Work out the finished part from the listing and answer in its coordinate system (mm). Face numbers are marked on the shaded views. A direction names the side the tool comes from. Round coordinates to 2 decimals unless told otherwise and drop trailing zeros. Write each loop counter-clockwise with the first axis right and the second up, starting at its lowest first coordinate (ties: lowest second). Pieces come first, ordered by that corner, then holes. Notation, with made-up numbers: M -21,53.25 L 5,53.25 A9 ccw 5,63.25 Z; hole C -26.5,48 d9. An arc over 180 degrees is marked long. One line per item, written item: value. Start each with the question number.
Q1. A tool of negligible diameter and unlimited length cuts with its end or side. For the marked faces 4 and 5, from which of +Z, -Z, +X, -X, +Y, -Y can it reach the whole face along a straight path? Write none if from no direction.
Q2. The mould has two halves that part along Y. Classify the marked faces 1, 2 and 3: released by +Y, released by -Y, zero draft, split by the parting line, or undercut.
Q3. Find section A-A (z = -3). Write down the section's boundary in (x, y), and give its area (3 significant figures).
Q4. Consider probe 1 along X at (y, z) = (-34, -2.25); probe 2 along Y at (x, z) = (8, 3.25). Determine where each line is inside the solid, lowest interval first.
Q5. Find section B-B (x = -14). Write down the section's boundary in (y, z), and give its area (3 significant figures).
Q6. Find section C-C (y = -24). Write down the section's boundary in (x, z), and give its area (3 significant figures).
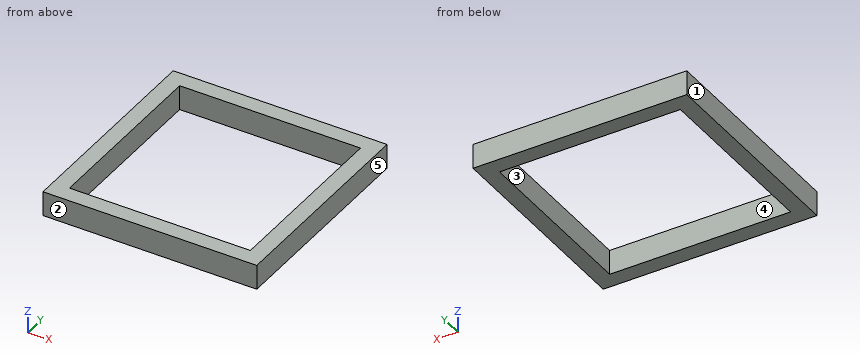
from build123d import *

# Parameters (mm, degrees)
SKETCH_W     = 65
SKETCH_H     = 65
PAD_DEPTH    = 3.75
SKETCH001_W  = 55
SKETCH001_H  = 55
POCKET_DEPTH = 7.501


with BuildPart() as part:
    # Sketch → Pad (new body, symmetric)
    with BuildSketch(Plane.XY):
        with Locations((-6.193032, -10.750862)):
            Rectangle(SKETCH_W, SKETCH_H)
    extrude(amount=PAD_DEPTH, both=True)

    # Sketch001 (on Face5 of Pad) → Pocket (cut, through all)
    with BuildSketch(Plane(origin=(0, 0, -3.75), x_dir=(1, 0, 0), z_dir=(0, 0, -1))):
        with Locations((-6.193032, 10.750862)):
            Rectangle(SKETCH001_W, SKETCH001_H)
    extrude(amount=-POCKET_DEPTH, mode=Mode.SUBTRACT)


solid = part.part
The answers:
1. face 4: +Z, -Z
1. face 5: +Z, -Z, +X, +Y, -Y
2. face 1: zero draft
2. face 2: released by -Y
2. face 3: undercut
3. outline: M -38.69,-43.25 L 26.31,-43.25 L 26.31,21.75 L -38.69,21.75 Z; hole M -33.69,-38.25 L 21.31,-38.25 L 21.31,16.75 L -33.69,16.75 Z
3. area: 1,200 mm2
4. probe 1: -38.69 to -33.69, 21.31 to 26.31
4. probe 2: -43.25 to -38.25, 16.75 to 21.75
5. outline: M -43.25,-3.75 L -38.25,-3.75 L -38.25,3.75 L -43.25,3.75 Z; M 16.75,-3.75 L 21.75,-3.75 L 21.75,3.75 L 16.75,3.75 Z
5. area: 75.0 mm2
6. outline: M -38.69,-3.75 L -33.69,-3.75 L -33.69,3.75 L -38.69,3.75 Z; M 21.31,-3.75 L 26.31,-3.75 L 26.31,3.75 L 21.31,3.75 Z
6. area: 75.0 mm2
